Autodesk Inventor part; units mm, degrees
ref_plane "YZ Plane" through (0, 0, 0) normal (1, 0, 0) x (0, 1, 0)
ref_plane "XZ Plane" through (0, 0, 0) normal (0, 1, 0) x (-1, 0, 0)
ref_plane "XY Plane" through (0, 0, 0) normal (0, 0, 1) x (1, 0, 0)
sketch "Эскиз1" plane through (0, 0, 0) normal (0, 0, 1) x (1, 0, 0)
  line L0 (-41.7, -37.7) -> (-41.7, -22.5)
  line L1 (-41.7, -22.5) -> (-37.5, -22.5)
  line L2 (-37.5, -22.5) -> (-37.5, -24.2)
  line L3 (-37.5, -24.2) -> (-27.2, -24.2)
  line L4 (-27.2, -24.2) -> (-27.2, -22.5)
  line L5 (-27.2, -22.5) -> (-25, -22.5)
  line L6 (-25, -22.5) -> (-25, -24.2)
  line L7 (-25, -24.2) -> (-22.5, -24.2)
  line L8 (-22.5, -24.2) -> (-22.5, -61.2)
  line L9 (-22.5, -61.2) -> (-25, -61.2)
  line L10 (-25, -61.2) -> (-25, -62.9)
  line L11 (-25, -62.9) -> (-40, -62.9)
  line L12 (-40, -62.9) -> (-40, -55.0851)
  line L13 (-44.2, -20) -> (-20, -20)
  line L14 (-20, -20) -> (-20, -65.4)
  line L15 (-60, -70) -> (-20, -70)
  line L16 (-20, -65.4) -> (-42.5, -65.4)
  line L17 (-41.7, -37.7) -> (-55.2, -37.7)
  line L18 (-44.2, -20) -> (-44.2, -29.7)
  line L19 (-55.2, -37.7) -> (-55.2, -44.1)
  line L20 (-44.2, -29.7) -> (-57.7, -35.2)
  line L21 (-57.7, -35.2) -> (-57.7, -46.6)
  line L22 (-60, -20) -> (-60, -70)
  line L23 (-42.5, -65.4) -> (-42.5, -54.6)
  line L24 (-55.2, -44.1) -> (-53.2, -44.1)
  line L25 (-53.2, -44.1) -> (-53.2, -46.6)
  line L26 (-53.2, -46.6) -> (-57.7, -46.6)
  line L27 (-49.2, -44.1) -> (-49.2, -46.6)
  line L28 (-49.2, -46.6) -> (-42.5, -54.6)
  line L29 (-49.2, -44.1) -> (-40, -55.0851)
  line L30 (-49.2, -44.1) -> (-46.2, -44.1)
  line L31 (-46.2, -44.1) -> (-46.2, -47.6821)
  line L32 (-25, -62.9) -> (-22.5, -65.4)
  line L33 (-30, -62.9) -> (-32.5, -65.4)
  line L34 (-46.2, -44.1) -> (-46.2, -37.7)
  line L35 (-20, -70) -> (-20, -20)
  line L36 (-20, -20) -> (-60, -20)
  line L37 (-53.2, -46.6) -> (-49.2, -46.6)
  line L38 (-53.2, -44.1) -> (-55.7, -46.6)
  line L39 (-49.2, -44.1) -> (-46.7, -49.5851)
  circle A0 centre (-54.1298, -30.506) radius 0.8
  circle A1 centre (-54.1298, -30.506) radius 3
  line L40 (-55.7762, -34.4162) -> (-56.908, -31.6379)
  line L41 (-50.2196, -32.1524) -> (-51.3515, -29.3742)
  circle A2 centre (-33.7426, -62.4) radius 0.8
  circle A3 centre (-33.7426, -62.4) radius 3
  line L42 (-29, -50.4) -> (-26, -50.4)
  line L43 (-26, -50.4) -> (-26, -60.4)
  line L44 (-26, -60.4) -> (-29, -60.4)
  line L45 (-29, -60.4) -> (-29, -50.4)
  circle A4 centre (-44.2, -35.2) radius 0.8
  circle A5 centre (-44.2, -35.2) radius 3
  line L46 (-40.5725, -65.4) -> (-42.5, -58.2063)
  point P0 (0, 0)
  point P1 (-44.2, -20)
  point P2 (-42.5417, -37.7)
  point P3 (-41.7, -36.8583)
  point P4 (-41.7, -33.5417)
  point P5 (-45.8583, -37.7)
  dimension "d0" = 16.7
  dimension "d1" = 4.2
  dimension "d2" = 2.2
  dimension "d3" = 1.7
  dimension "d4" = 40.4
  dimension "d5" = 1.7
  dimension "d6" = 2.5
  dimension "d7" = 15
  dimension "d8" = 2.5
  dimension "d9" = 2.5
  dimension "d10" = 2.5
  dimension "d11" = 15.2
  dimension "d12" = 2.5
  dimension "d14" = 2.5
  dimension "d15" = 2.5
  dimension "d16" = 8
  dimension "d17" = 2.5
  dimension "d18" = 6.4
  dimension "d19" = 2.5
  dimension "d20" = 2
  dimension "d21" = 4
  dimension "d22" = 2.5
  dimension "d23" = 3
  dimension "d24" = 5
  dimension "d25" = 2.5
  dimension "d26" = 8
  dimension "d27" = 2.5
  dimension "d28" = 2.5
  dimension "d29" = 2.5
  dimension "d30" = 20
  dimension "d31" = 20
  dimension "d32" = 50
  dimension "d33" = 40
  dimension "d44" = 37.7
  dimension "d55" = 1.6
  dimension "d57" = 6
  dimension "d58" = 6.5
  dimension "d60" = 1.6
  dimension "d61" = 6
  dimension "d66" = 6
  dimension "d67" = 9
  dimension "d68" = 5
  dimension "d69" = 15
  dimension "d77" = 1.6
  dimension "d78" = 6
  dimension "d80" = 15.2
  dimension "d81" = 24.2
  dimension "d83" = 15
  dimension "d84" = 1.2
extrude "Выдавливание1" add sketch "Эскиз1" along normal blind 2.5 contours L17 A5 L0 | L0 A5 L1 L2 L3 L4 L5 L6 L7 L8 L9 L10 L11 A3 L12 L29 L31 L34 L17 | A5 L17 L0 | L0 A5 | A5 L17 | A5 L17 L19 L24 L38 L26 L21 L20 L18 L13 L14 L16 L32 L10 L9 L8 L7 L6 L5 L4 L3 L2 L1 L0 | L34 L30 L27 L37 L25 L24 L19 L17 | L31 L29 L30 | L39 L28 L27 | L29 L12 L11 A3 L16 L46 L23 L28 L39 | L25 L26 L38 | A3 L11 A2 | L11 A2 A3 | A3 L33 L16 | L11 L33 A3 | L33 L11 L32 L16 | L42 L43 L44 L45
extrude "Выдавливание3" add sketch "Эскиз1" against normal blind 7 contours L33 L11 L32 L16
chamfer "Фаска1" distance 2.5 angle 45 1 edges at (-27.5, -65.4, -7)
fillet "Сопряжение1" radius 2 12 edges at (-44.2, -24.85, 2.5) (-50.95, -32.45, 2.5) (-57.7, -40.9, 2.5) (-53.45, -46.6, 2.5) (-45.85, -50.6, 2.5) (-42.5, -56.4032, 2.5) (-30.2862, -65.4, 2.5) (-57.7, -46.6, 1.25) (-57.7, -35.2, 1.25) (-32.1, -20, 2.5) (-44.2, -20, 1.25) (-41.5362, -61.8032, 2.5)
extrude "Выдавливание4" cut sketch "Эскиз1" against normal blind 0.5 from surface at 2.5 contours A5 L17 L0 | L0 A5 | A5 L17 | A3 L11 A2 | L11 A2 A3 picked at (-44.1679, -37.1314)
extrude "Выдавливание5" cut sketch "Эскиз1" along normal blind 1.5 contours L42 L43 L44 L45
fillet "Сопряжение3" radius 1 4 edges at (-29, -55.4, 0) (-27.5, -50.4, 0) (-26, -55.4, 0) (-27.5, -60.4, 0)
fillet "Сопряжение4" radius 3 2 edges at (-40.5725, -65.4, 0.25) (-40.123, -64.8142, 1.9142)
properties part number "Top_3DПЕЧАТЬ"
Input: part model. Units: mm. Frame: model coordinates. A direction names the side the tool comes from. Give positions to 0.01 mm unless a question says otherwise; leave off trailing zeros. Order: outer loops, then holes, each group sorted by start corner. A loop starts at its lowest first (then second) coordinate and runs counter-clockwise, first axis right, second up. Notation, with made-up numbers: (-25.5, -14.75) - (-10.5, -14.75) arc R22 cw to (-10.5, 12.25) - close; hole circle Ø1 at (-12.75, -18.75). An arc over 180 degrees is marked (long way). One line per item, written item: value.
1. Reachability of faces 1 (the face through (-27, -62.9, -3)), 2 (the face through (-33.92, -61.62, 0.99)), 3 (the face through (-34, -61, 2)), 4 (the face through (-31.2, -64.1, -2.7)), 5 (the face through (-29.285, -55.316, 0.301)) from +Z, -Z, +X, -X, +Y, -Y: full face, straight path, thin tool, end or side. Return the list, or none.
Determined:
face 1: -Z, +X, -X, +Y
face 2: +Z, -Z
face 3: +Z
face 4: -Z, -X, +Y
face 5: -Z
2. Line query: probe 1 along Z at (x, y) = (-38.5, -34); probe 2 along Y at (x, z) = (-28.5, -0.75); probe 3 along X at (y, z) = (-62.4, 2.2). Output: solid intervals per line, ascending.
Determined:
probe 1: 0 to 2.5
probe 2: -65.4 to -62.9
probe 3: -40.4 to -36.74, -30.74 to -20
3. Cut plane B-B, the plane z = -4. Output: boundary loops of the cut face in (x, y).
Determined:
outline: (-32.5, -65.4) - (-22.5, -65.4) - (-25, -62.9) - (-30, -62.9) - close
4. Pin query (flat end, axial travel): pin 1 Ø3 at (x, z) = (-28.5, -2.5) entering from +Y; pin 2 Ø0.9 at (x, y) = (-28, -53.5) entering from -Z; pin 3 Ø2 at (x, z) = (-32.5, -2.5) entering from +Y; pin 4 Ø1 at (x, y) = (-44.2, -35.2) entering from -Z. Return the tip coordinate at first contact, or that it passes through.
Determined:
pin 1: y = -62.9
pin 2: z = 1.5
pin 3: y = -64.4
pin 4: through
5. Draft query along X for faces 6 (the face through (-27.6, -64.4, -5.5)), 7 (the face through (-44, -34, 2)), 8 (the face through (-41.825, -60.726, 0.246)). Return one class per face: released by +X, released by -X, zero draft, split by the parting line, or undercut.
Determined:
face 6: zero draft
face 7: undercut
face 8: released by -X
